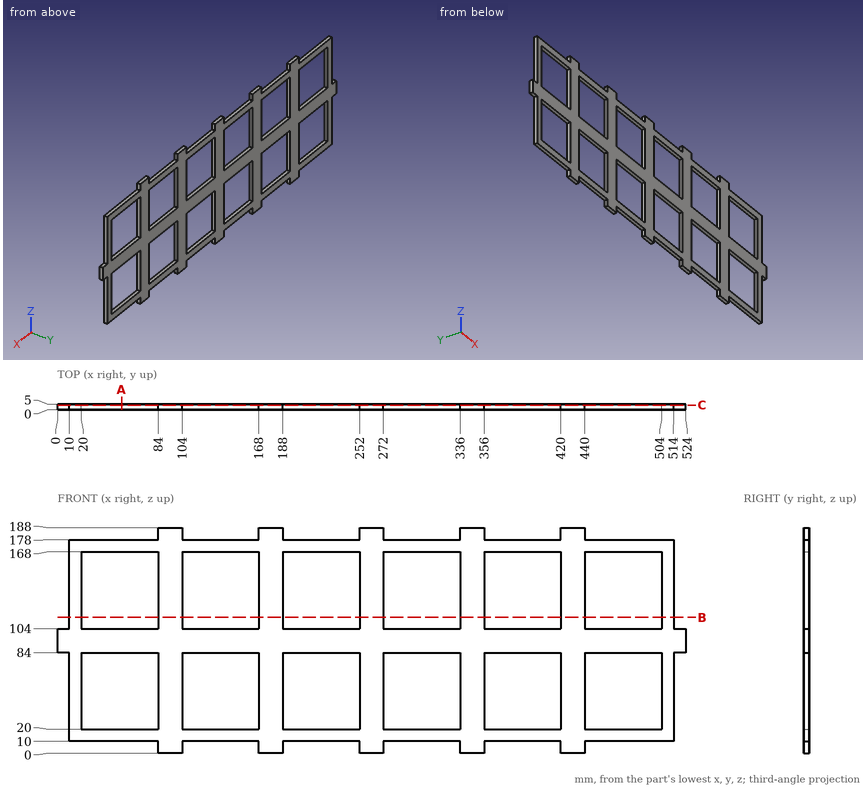
Here's the drawing with two shaded views (mm, measured from the low corner). I have some questions. Round coordinates to 2 decimals unless told otherwise and drop trailing zeros. Loops run counter-clockwise (first coordinate to the right, second up) from the corner with the lowest first, then second, coordinate; pieces in that order, holes last. Notation, with made-up numbers: (-17.75, -37) - (-6.75, -37) arc R18 cw to (-6.75, -24) - close; hole circle Ø7 at (14, 15). An arc over 180 degrees is marked (long way). Write item = value, one per line.
1) Imagine slicing it at A-A (x = 53.5). Please give me the cut outline in (y, z).
Computed:
outline = (0, 10) - (5, 10) - (5, 20) - (0, 20) - close; (0, 84) - (5, 84) - (5, 104) - (0, 104) - close; (0, 168) - (5, 168) - (5, 178) - (0, 178) - close
2) I need wall thicknesses on line 1 along Z through (x, y) = (419.5, 1.85); line 2 along X through (y, z) = (4.4, 9). Which ranges of each line are inside material? Lowest first, please. Write a range as from..to.
Computed:
line_1 = 10..20, 84..104, 168..178
line_2 = 84..104, 168..188, 252..272, 336..356, 420..440
3) Imagine slicing it at B-B (z = 113.5). Please give me the cut outline in (x, y).
Computed:
outline = (10, 0) - (20, 0) - (20, 5) - (10, 5) - close; (84, 0) - (104, 0) - (104, 5) - (84, 5) - close; (168, 0) - (188, 0) - (188, 5) - (168, 5) - close; (252, 0) - (272, 0) - (272, 5) - (252, 5) - close; (336, 0) - (356, 0) - (356, 5) - (336, 5) - close; (420, 0) - (440, 0) - (440, 5) - (420, 5) - close; (504, 0) - (514, 0) - (514, 5) - (504, 5) - close
4) Imagine slicing it at C-C (y = 4.15). Give the number of separate pieces and of enclosed holes in the cut face, and give its area (3 significant figures).
Computed:
separate_pieces = 1
enclosed_holes = 12
area = 37,900 mm2
5) I'm going to push flat-ended pins straight in: P1, Ø2.5, axis at y = 1.5, z = 41.5, coming from the -X side; P2, Ø1.5, axis at x = 443, y = 2.5, coming from the +Z side; P3, Ø2.5, axis at y = 2.5, z = 56.5, coming from the +X side. Where does each tip first touch, or does it pass through?
Computed:
P1 = 10
P2 = 178
P3 = 514
